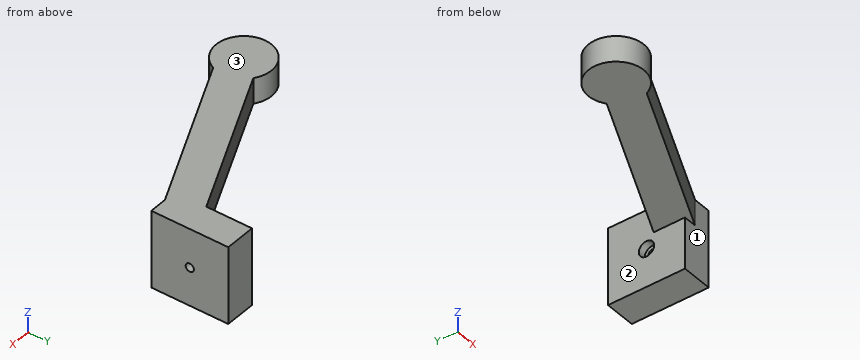
```python
from build123d import *

# Parameters (mm, degrees)
SKETCH_W        = 12
SKETCH_H        = 30
PAD_DEPTH       = 30
PAD001_DEPTH    = 10
SKETCH002_R     = 10.776267
PAD002_DEPTH    = 10
SKETCH004_R     = 3
POCKET001_DEPTH = 3
SKETCH005_R     = 1.6
POCKET_DEPTH    = 9.001


with BuildPart() as part:
    # Sketch → Pad (new body)
    with BuildSketch(Plane.XY):
        Rectangle(SKETCH_W, SKETCH_H)
    extrude(amount=PAD_DEPTH)

    # Sketch001 → Pad001 (join)
    with BuildSketch(Plane.XY.offset(30)):
        Polygon((0, 0), (-73.854295, -34.438823), (-73.854295, -49.021726), (0, -14.582903), align=None)
    extrude(amount=-PAD001_DEPTH)

    # Sketch002 → Pad002 (join)
    with BuildSketch(Plane.XY.offset(30)):
        with Locations((-72.459145, -39.435551)):
            Circle(SKETCH002_R)
    extrude(amount=-PAD002_DEPTH)

    # Sketch004 → Pocket001 (cut)
    with BuildSketch(Plane.YZ.offset(-6)):
        with Locations((0, 14.871989)):
            Circle(SKETCH004_R)
    extrude(amount=POCKET001_DEPTH, mode=Mode.SUBTRACT)

    # Sketch005 → Pocket (cut, through all)
    with BuildSketch(Plane.YZ.offset(-3)):
        with Locations((0, 14.898449)):
            Circle(SKETCH005_R)
    extrude(amount=POCKET_DEPTH, mode=Mode.SUBTRACT)


solid = part.part
```
Design review of the part built by this model. Coordinates are the model's own, in mm. Face numbers are marked on the shaded views. A direction names the side the tool comes from. Give positions to 0.01 mm unless a question says otherwise; leave off trailing zeros. Order: outer loops, then holes, each group sorted by start corner. A loop starts at its lowest first (then second) coordinate and runs counter-clockwise, first axis right, second up. Notation, with made-up numbers: (3.5, 4) -> (60.5, 4) arc R19 cw to (60.5, 31) -> close; hole circle Ø3 at (44, -9.75). An arc over 180 degrees is marked (long way). Write each question's results on one line, items separated by ' | '. Start each with the question number.
Q1. Add section B-B on z = 24.75. Give the boundary of the cut face in (x, y), and give its area (3 significant figures).
Q2. Add section D-D on x = -70. Give the boundary of the cut face in (y, z).
Q3. Wall thickness on L1, parallel to Z at x = 2.25, y = 0; L2, parallel to Z at x = -4.1, y = 0; L3, parallel to X at y = 2, z = 7.5: over which ranges is each line inside the solid? List them lowest first. Write a range as from..to.
Q4. Machinability: for the marked faces 1, 2 and 3, which of the approach directions +Z, -Z, +X, -X, +Y, -Y give a long, thin tool a straight path to every point of the face, cutting with its end or side? Answer none if there is none.
Q5. Add section C-C on y = 10.5. Give the boundary of the cut face in (x, z), and give its area (3 significant figures).
Q6. Add section A-A on y = 0. Give the boundary of the cut face in (x, z).
Q7. For pin 1 (5 mm diameter, centred on x = -40, z = 22.5, fed in from -Y); pin 2 (8 mm diameter, centred on y = 0, z = 14.87, fed in from -X); pin 3 (1 mm diameter, centred on x = -54.5, y = -31.5, fed in from -Z), all flat-tipped, find the tip position at first contact; note any pin that passes through.
Found:
1) outline: (-66.03, -30.79) arc R10.78 ccw (long way) to (-62.59, -43.77) -> (-0.89, -15) -> (6, -15) -> (6, 15) -> (-6, 15) -> (-6, -2.8) -> close | area: 1,560 mm2
2) outline: (-49.93, 20) -> (-28.94, 20) -> (-28.94, 30) -> (-49.93, 30) -> close
3) L1: z = 0..13.3, 16.5..30 | L2: z = 0..11.87, 17.87..30 | L3: x = -6..6
4) face 1: -Z, +X, -Y | face 2: -Z, -X, +Y | face 3: +Z, +X, -X, +Y, -Y
5) outline: (-6, 0) -> (6, 0) -> (6, 30) -> (-6, 30) -> close | area: 360 mm2
6) outline: (-6, 0) -> (6, 0) -> (6, 13.3) -> (-3, 13.3) -> (-3, 11.87) -> (-6, 11.87) -> close; (-6, 17.87) -> (-3, 17.87) -> (-3, 16.5) -> (6, 16.5) -> (6, 30) -> (-6, 30) -> close
7) pin 1: stops at y = -34.4 | pin 2: stops at x = -6 | pin 3: stops at z = 20
